Check sheet for the modelled part. Datum: model origin and axes. Units: mm. Give positions to 0.01 mm unless a question says otherwise; leave off trailing zeros. Order: outer loops, then holes, each group sorted by start corner. A loop starts at its lowest first (then second) coordinate and runs counter-clockwise, first axis right, second up. Notation, with made-up numbers: M 37,85.25 L 87,85.25 A18 ccw 87,105.25 Z; hole C -15,67 d7. An arc over 180 degrees is marked long. Answer in a Markdown table with one row per item. Add a question column.
from build123d import *

# Parameters (mm, degrees)
SKETCH_W   = 30
SKETCH_H   = 20
SKETCH_R   = 1.5
SKETCH_W_2 = 4
SKETCH_H_2 = 7
PAD_DEPTH  = 3


with BuildPart() as part:
    # Sketch → Pad (new body)
    with BuildSketch(Plane.XY):
        with Locations((15, 10)):
            Rectangle(SKETCH_W, SKETCH_H)
        with Locations((5, 8)):
            Circle(SKETCH_R, mode=Mode.SUBTRACT)
        with Locations((11, 15)):
            Circle(SKETCH_R, mode=Mode.SUBTRACT)
        with Locations((11, 6)):
            Circle(SKETCH_R, mode=Mode.SUBTRACT)
        with Locations((5, 13)):
            Circle(SKETCH_R, mode=Mode.SUBTRACT)
        with Locations((5, 3)):
            Circle(SKETCH_R, mode=Mode.SUBTRACT)
        with Locations((22, 8)):
            Rectangle(SKETCH_W_2, SKETCH_H_2, mode=Mode.SUBTRACT)
    pad = extrude(amount=PAD_DEPTH)

    # Mirrored: Pad across face of Pad
    add(pad.mirror(Plane(origin=(30, 10, 1.5), x_dir=(0, 1, 0), z_dir=(1, 0, 0))))


solid = part.part
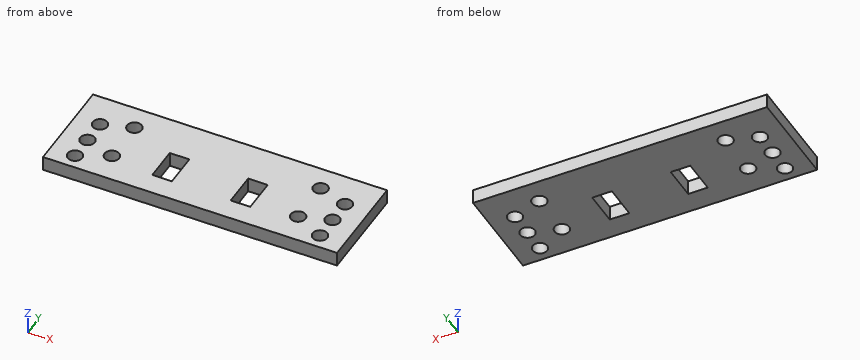
Q1. Cross-section at C-C (x = 49). Record the boundary of the cut face in (y, z), and give its area (3 significant figures).
Q2. Cross-section at A-A (x = 55). Record the boundary of the cut face in (y, z).
Q3. Go/stop test with flat-tipped pins: pin 1 (2.5 mm diameter, centred on x = 5, y = 8, fed in from -Z); pin 2 (4 mm diameter, centred on x = 21.5, y = 3, fed in from -Z). Record where each tip stops, or that it passes through.
Q4. Cross-section at D-D (x = 23). Record the boundary of the cut face in (y, z), and give its area (3 significant figures).
Q5. Thickness scan on probe 1 along Y at (x, z) = (49, 1.4); probe 2 along Y at (x, z) = (5, 1.6); probe 3 along X at (y, z) = (14, 0.7). Record the ranges inside material, lowest first.
Q6. Cross-section at B-B (z = 1.3). State how many separate pieces and enclosed holes the cut face has, and give its area (3 significant figures).
Values follow:
| question | item | result |
|---|---|---|
| 1 | outline | M 0,0 L 4.5,0 L 4.5,3 L 0,3 Z; M 7.5,0 L 13.5,0 L 13.5,3 L 7.5,3 Z; M 16.5,0 L 20,0 L 20,3 L 16.5,3 Z |
| 1 | area | 42.0 mm² |
| 2 | outline | M 0,0 L 1.5,0 L 1.5,3 L 0,3 Z; M 4.5,0 L 6.5,0 L 6.5,3 L 4.5,3 Z; M 9.5,0 L 11.5,0 L 11.5,3 L 9.5,3 Z; M 14.5,0 L 20,0 L 20,3 L 14.5,3 Z |
| 3 | pin 1 | through |
| 3 | pin 2 | z = 0 |
| 4 | outline | M 0,0 L 4.5,0 L 4.5,3 L 0,3 Z; M 11.5,0 L 20,0 L 20,3 L 11.5,3 Z |
| 4 | area | 39.0 mm² |
| 5 | probe 1 | 0 to 4.5, 7.5 to 13.5, 16.5 to 20 |
| 5 | probe 2 | 0 to 1.5, 4.5 to 6.5, 9.5 to 11.5, 14.5 to 20 |
| 5 | probe 3 | 0 to 3.88, 6.12 to 9.88, 12.12 to 47.88, 50.12 to 53.88, 56.12 to 60 |
| 6 | separate pieces | 1 |
| 6 | enclosed holes | 12 |
| 6 | area | 1,070 mm² |
